```python
from build123d import *

# Parameters (mm, degrees)
F0_R         = 15.113
F1_DEPTH     = 16.51
F2_DEPTH     = 1.905
F3_T1_DEPTH  = 63.5
F3_T3_DEPTH  = 63.5
F3_T6_ANGLE  = 90
F3_T8_ANGLE  = 90
F3_T10_ANGLE = 90
F3_T12_ANGLE = 90
F3_T14_ANGLE = 90
F3_T16_ANGLE = 90
F3_T18_ANGLE = 90
F3_T20_ANGLE = 90


# Not quite as in the source:
# - a fillet or chamfer that OpenCascade refuses, or shapes differently, is made with other operations: its cross-section is extruded or revolved along the edge and cut away or added


with BuildPart() as f1:
    # F0 (on Top) → F1 (new body)
    with BuildSketch(Plane.XY):
        with BuildLine():
            Line((31.75, 44.45), (-31.75, 44.45))
            ThreePointArc((-31.75, 44.45), (-40.7302561211, 40.7302561211), (-44.45, 31.75))
            Line((-44.45, 31.75), (-44.45, -31.75))
            ThreePointArc((-44.45, -31.75), (-40.7302561211, -40.7302561211), (-31.75, -44.45))
            Line((-31.75, -44.45), (31.75, -44.45))
            ThreePointArc((31.75, -44.45), (40.7302561211, -40.7302561211), (44.45, -31.75))
            Line((44.45, -31.75), (44.45, 31.75))
            ThreePointArc((44.45, 31.75), (40.7302561211, 40.7302561211), (31.75, 44.45))
        make_face()
        with Locations((-22.225, -22.225)):
            Circle(F0_R, mode=Mode.SUBTRACT)
        with Locations((22.225, -22.225)):
            Circle(F0_R, mode=Mode.SUBTRACT)
        with BuildLine():
            ThreePointArc((-6.9787090866, 24.098385063), (-6.8187195919, 22.8373692451), (-6.7652637085, 21.5673692451))
            ThreePointArc((-6.7652637085, 21.5673692451), (-6.8187195919, 20.2973692451), (-6.9787090866, 19.0363534272))
            ThreePointArc((-6.9787090866, 19.0363534272), (-11.1917589244, 10.880864461), (-19.3472478905, 6.6678146232))
            ThreePointArc((-19.3472478905, 6.6678146232), (-21.8782637085, 6.4543692451), (-24.4092795264, 6.6678146232))
            ThreePointArc((-24.4092795264, 6.6678146232), (-32.5647684925, 10.880864461), (-36.7778183303, 19.0363534272))
            ThreePointArc((-36.7778183303, 19.0363534272), (-36.9912637085, 21.5673692451), (-36.7778183303, 24.098385063))
            ThreePointArc((-36.7778183303, 24.098385063), (-32.5647684925, 32.2538740292), (-24.4092795264, 36.4669238669))
            ThreePointArc((-24.4092795264, 36.4669238669), (-21.8782637085, 36.6803692451), (-19.3472478905, 36.4669238669))
            ThreePointArc((-19.3472478905, 36.4669238669), (-11.1917589244, 32.2538740292), (-6.9787090866, 24.098385063))
        make_face(mode=Mode.SUBTRACT)
        with Locations((22.225, 22.225)):
            Circle(F0_R, mode=Mode.SUBTRACT)
    extrude(amount=F1_DEPTH)

    # F0 (on Top) → F2 (join)
    with BuildSketch(Plane.XY):
        with BuildLine():
            ThreePointArc((-6.9787090866, 19.0363534272), (-6.8187195919, 20.2973692451), (-6.7652637085, 21.5673692451))
            ThreePointArc((-6.7652637085, 21.5673692451), (-6.8187195919, 22.8373692451), (-6.9787090866, 24.098385063))
            Line((-6.9787090866, 24.098385063), (-19.3472478905, 23.9739259511))
            ThreePointArc((-19.3472478905, 23.9739259511), (-18.6350300602, 22.8631283867), (-18.3857637085, 21.5673692451))
            ThreePointArc((-18.3857637085, 21.5673692451), (-18.668711127, 20.1902968152), (-19.4717070024, 19.0363534272))
            Line((-19.4717070024, 19.0363534272), (-6.9787090866, 19.0363534272))
        make_face()
        with BuildLine():
            Line((-19.3472478905, 23.9739259511), (-19.3472478905, 36.4669238669))
            ThreePointArc((-19.3472478905, 36.4669238669), (-21.8782637085, 36.6803692451), (-24.4092795264, 36.4669238669))
            Line((-24.4092795264, 36.4669238669), (-24.4092795264, 23.9739259511))
            ThreePointArc((-24.4092795264, 23.9739259511), (-21.8782637085, 25.0598692451), (-19.3472478905, 23.9739259511))
        make_face()
        with BuildLine():
            ThreePointArc((-18.3857637085, 21.5673692451), (-18.6350300602, 22.8631283867), (-19.3472478905, 23.9739259511))
            ThreePointArc((-19.3472478905, 23.9739259511), (-21.8782637085, 25.0598692451), (-24.4092795264, 23.9739259511))
            ThreePointArc((-24.4092795264, 23.9739259511), (-25.3707637085, 21.5673692451), (-24.4092795264, 19.160812539))
            ThreePointArc((-24.4092795264, 19.160812539), (-21.9662695904, 18.0759782308), (-19.4717070024, 19.0363534272))
            ThreePointArc((-19.4717070024, 19.0363534272), (-18.668711127, 20.1902968152), (-18.3857637085, 21.5673692451))
        make_face()
        with BuildLine():
            ThreePointArc((-24.4092795264, 19.160812539), (-25.3707637085, 21.5673692451), (-24.4092795264, 23.9739259511))
            Line((-24.4092795264, 23.9739259511), (-36.7778183303, 24.098385063))
            ThreePointArc((-36.7778183303, 24.098385063), (-36.9912637085, 21.5673692451), (-36.7778183303, 19.0363534272))
            Line((-36.7778183303, 19.0363534272), (-24.4092795264, 19.160812539))
        make_face()
        with BuildLine():
            ThreePointArc((-24.4092795264, 6.6678146232), (-21.8782637085, 6.4543692451), (-19.3472478905, 6.6678146232))
            Line((-19.3472478905, 6.6678146232), (-19.4717070024, 19.0363534272))
            ThreePointArc((-19.4717070024, 19.0363534272), (-21.9662695904, 18.0759782308), (-24.4092795264, 19.160812539))
            Line((-24.4092795264, 19.160812539), (-24.4092795264, 6.6678146232))
        make_face()
    extrude(amount=F2_DEPTH)

    # F3: fillet of radius 8.255 on 3 edges, made by hand

    # F3_s2 → F3_t1 (cut)
    with BuildSketch(Plane.XZ.offset(-31.75)):
        with BuildLine():
            ThreePointArc((-36.195, 16.51), (-42.0321664787, 14.0921664787), (-44.45, 8.255))
            Line((-44.45, 8.255), (-44.45, 16.51))
            Line((-44.45, 16.51), (-36.195, 16.51))
        make_face()
        with BuildLine():
            ThreePointArc((36.195, 0), (42.0321664787, 2.4178335213), (44.45, 8.255))
            Line((44.45, 8.255), (44.45, 0))
            Line((44.45, 0), (36.195, 0))
        make_face()
        with BuildLine():
            ThreePointArc((-36.195, 0), (-42.0321664787, 2.4178335213), (-44.45, 8.255))
            Line((-44.45, 8.255), (-44.45, 0))
            Line((-44.45, 0), (-36.195, 0))
        make_face()
        with BuildLine():
            ThreePointArc((36.195, 16.51), (42.0321664787, 14.0921664787), (44.45, 8.255))
            Line((44.45, 8.255), (44.45, 16.51))
            Line((44.45, 16.51), (36.195, 16.51))
        make_face()
    extrude(amount=F3_T1_DEPTH, mode=Mode.SUBTRACT)

    # F3_s4 → F3_t3 (cut)
    with BuildSketch(Plane.YZ.offset(-31.75)):
        with BuildLine():
            ThreePointArc((-36.195, 0), (-42.0321664787, 2.4178335213), (-44.45, 8.255))
            Line((-44.45, 8.255), (-44.45, 0))
            Line((-44.45, 0), (-36.195, 0))
        make_face()
        with BuildLine():
            ThreePointArc((44.45, 8.255), (42.0321664787, 2.4178335213), (36.195, 0))
            Line((36.195, 0), (44.45, 0))
            Line((44.45, 0), (44.45, 8.255))
        make_face()
        with BuildLine():
            ThreePointArc((-36.195, 16.51), (-42.0321664787, 14.0921664787), (-44.45, 8.255))
            Line((-44.45, 8.255), (-44.45, 16.51))
            Line((-44.45, 16.51), (-36.195, 16.51))
        make_face()
        with BuildLine():
            ThreePointArc((44.45, 8.255), (42.0321664787, 14.0921664787), (36.195, 16.51))
            Line((36.195, 16.51), (44.45, 16.51))
            Line((44.45, 16.51), (44.45, 8.255))
        make_face()
    extrude(amount=F3_T3_DEPTH, mode=Mode.SUBTRACT)

    # F3_s5 → F3_t6 (revolve, cut)
    with BuildSketch(Plane.YZ.offset(-31.75)):
        with BuildLine():
            ThreePointArc((44.45, 8.255), (42.0321664787, 14.0921664787), (36.195, 16.51))
            Line((36.195, 16.51), (44.45, 16.51))
            Line((44.45, 16.51), (44.45, 8.255))
        make_face()
    revolve(axis=Axis((-31.75, 31.75, 16.51), (0, 0, 1)), revolution_arc=F3_T6_ANGLE, mode=Mode.SUBTRACT)

    # F3_s7 → F3_t8 (revolve, cut)
    with BuildSketch(Plane.XZ.offset(31.75)):
        with BuildLine():
            ThreePointArc((-36.195, 0), (-42.0321664787, 2.4178335213), (-44.45, 8.255))
            Line((-44.45, 8.255), (-44.45, 0))
            Line((-44.45, 0), (-36.195, 0))
        make_face()
    revolve(axis=Axis((-31.75, -31.75, 0), (0, 0, 1)), revolution_arc=F3_T8_ANGLE, mode=Mode.SUBTRACT)

    # F3_s9 → F3_t10 (revolve, cut)
    with BuildSketch(Plane.YZ.offset(31.75)):
        with BuildLine():
            ThreePointArc((-36.195, 0), (-42.0321664787, 2.4178335213), (-44.45, 8.255))
            Line((-44.45, 8.255), (-44.45, 0))
            Line((-44.45, 0), (-36.195, 0))
        make_face()
    revolve(axis=Axis((31.75, -31.75, 0), (0, 0, 1)), revolution_arc=F3_T10_ANGLE, mode=Mode.SUBTRACT)

    # F3_s11 → F3_t12 (revolve, cut)
    with BuildSketch(Plane.XZ.offset(-31.75)):
        with BuildLine():
            ThreePointArc((44.45, 8.255), (42.0321664787, 2.4178335213), (36.195, 0))
            Line((36.195, 0), (44.45, 0))
            Line((44.45, 0), (44.45, 8.255))
        make_face()
    revolve(axis=Axis((31.75, 31.75, 0), (0, 0, 1)), revolution_arc=F3_T12_ANGLE, mode=Mode.SUBTRACT)

    # F3_s13 → F3_t14 (revolve, cut)
    with BuildSketch(Plane.YZ.offset(-31.75)):
        with BuildLine():
            ThreePointArc((44.45, 8.255), (42.0321664787, 2.4178335213), (36.195, 0))
            Line((36.195, 0), (44.45, 0))
            Line((44.45, 0), (44.45, 8.255))
        make_face()
    revolve(axis=Axis((-31.75, 31.75, 0), (0, 0, 1)), revolution_arc=F3_T14_ANGLE, mode=Mode.SUBTRACT)

    # F3_s15 → F3_t16 (revolve, cut)
    with BuildSketch(Plane.XZ.offset(31.75)):
        with BuildLine():
            ThreePointArc((-36.195, 16.51), (-42.0321664787, 14.0921664787), (-44.45, 8.255))
            Line((-44.45, 8.255), (-44.45, 16.51))
            Line((-44.45, 16.51), (-36.195, 16.51))
        make_face()
    revolve(axis=Axis((-31.75, -31.75, 16.51), (0, 0, 1)), revolution_arc=F3_T16_ANGLE, mode=Mode.SUBTRACT)

    # F3_s17 → F3_t18 (revolve, cut)
    with BuildSketch(Plane.YZ.offset(31.75)):
        with BuildLine():
            ThreePointArc((-36.195, 16.51), (-42.0321664787, 14.0921664787), (-44.45, 8.255))
            Line((-44.45, 8.255), (-44.45, 16.51))
            Line((-44.45, 16.51), (-36.195, 16.51))
        make_face()
    revolve(axis=Axis((31.75, -31.75, 16.51), (0, 0, 1)), revolution_arc=F3_T18_ANGLE, mode=Mode.SUBTRACT)

    # F3_s19 → F3_t20 (revolve, cut)
    with BuildSketch(Plane.XZ.offset(-31.75)):
        with BuildLine():
            ThreePointArc((44.45, 8.255), (42.0321664787, 14.0921664787), (36.195, 16.51))
            Line((36.195, 16.51), (44.45, 16.51))
            Line((44.45, 16.51), (44.45, 8.255))
        make_face()
    revolve(axis=Axis((31.75, 31.75, 16.51), (0, 0, 1)), revolution_arc=F3_T20_ANGLE, mode=Mode.SUBTRACT)


solid = f1.part
```
Work out the finished part from the listing and answer in its coordinate system (mm). A direction names the side the tool comes from. Give positions to 0.01 mm unless a question says otherwise; leave off trailing zeros. Loops run counter-clockwise (first coordinate to the right, second up) from the corner with the lowest first, then second, coordinate; pieces in that order, holes last. Notation, with made-up numbers: (49, 71) - (70, 71) arc R26 ccw to (70, 97) - close; hole circle Ø11 at (73, -36). An arc over 180 degrees is marked (long way). Use CSV: the item, a comma, the result in double quotes. Start each with the question number.
(1) Determine the mould class of faces 4 (the face through (-33, 33, 0)), 5 (the face through (-19.347, 30, 1)) for opening direction X: released by +X, released by -X, zero draft, split by the parting line, or undercut.
(2) A tool of negligible diameter and unlimited length cuts with its end or side. For faces 1 (the face through (-23, 22, 1.905)), 2 (the face through (-24.409, 13, 1)), 3 (the face through (33, 34, 16.51)), from which of +Z, -Z, +X, -X, +Y, -Y can it reach the whole face along a straight path? Write none if from no direction.
(3) Find section A-A, the plane x = 26.5. Determine the outline of the cut face in (y, z) (3 decimals).
(4) Find section D-D, the plane x = -12. Determine the outline of the cut face in (y, z) (3 decimals).
(5) Each of these flat-tipped pins is pushed along its axis until it touches: pin 1 (1 mm diameter, centred on y = 29.5, z = 1, fed in from +X); pin 2 (0.6 mm diameter, centred on y = 15.5, z = 0.5, fed in from -X); pin 3 (1 mm diameter, centred on y = 8, z = 14.5, fed in from +X); pin 4 (18 mm diameter, centred on x = 22.225, y = -22.225, fed in from -Z). Where does it stop, or does it pass through?
(6) Find section C-C, the plane y = 30. Determine the outline of the cut face in (x, z) (3 decimals).
(7) Find the intervals of material crossed by L1, parallel to Y at x = 16, z = 11.75; L2, parallel to X at y = 10.5, z = 10.5; L3, parallel to X at y = -12, z = 14, in increasing order.
(8) Find section B-B, the plane x = 3.5. Determine the outline of the cut face in (y, z) (3 decimals).
Results found:
1,face 4,"zero draft"
1,face 5,"undercut"
2,face 1,"+Z"
2,face 2,"+Z, -Z"
2,face 3,"+Z, +X, -X, +Y, -Y"
3,outline,"(-36.721, 0.017) - (-36.721, 16.493) arc R8.255 ccw to start; (-7.729, 0) - (7.729, 0) - (7.729, 16.51) - (-7.729, 16.51) - close; (36.721, 0.017) arc R8.255 ccw to (36.721, 16.493) - close"
4,outline,"(-36.195, 0) - (-33.354, 0) - (-33.354, 16.51) - (-36.195, 16.51) arc R8.255 ccw to start; (-11.096, 0) - (10.13, 0) - (10.13, 16.51) - (-11.096, 16.51) - close; (19.036, 0) - (24.048, 0) - (24.048, 1.905) - (19.036, 1.905) - close; (33.005, 0) - (36.195, 0) arc R8.255 ccw to (36.195, 16.51) - (33.005, 16.51) - close"
5,pin 1,"x = 40.94"
5,pin 2,"x = -39.74"
5,pin 3,"x = 42.12"
5,pin 4,"through"
6,outline,"(-36.195, 0) - (-34.42, 0) - (-34.42, 16.51) - (-36.195, 16.51) arc R8.255 ccw to start; (-24.409, 0) - (-19.347, 0) - (-19.347, 1.905) - (-24.409, 1.905) - close; (-9.337, 0) - (9.265, 0) - (9.265, 16.51) - (-9.337, 16.51) - close; (35.185, 0) - (36.195, 0) arc R8.255 ccw to (36.195, 16.51) - (35.185, 16.51) - close"
7,L1,"-43.67 to -36, -8.45 to 8.45, 36 to 43.67"
7,L2,"-44.14 to -32.17, -11.59 to 12.69, 31.76 to 44.14"
7,L3,"-42.12 to -33.35, -11.1 to 11.1, 33.35 to 42.12"
8,outline,"(-36.195, 0) - (36.195, 0) arc R8.255 ccw to (36.195, 16.51) - (-36.195, 16.51) arc R8.255 ccw to start"
